from build123d import *

# Parameters (mm, degrees)
F1_DEPTH  = 90
F2_T      = -1.5
F4_DEPTH  = 90.001
F6_DEPTH  = 90
F8_DEPTH  = 90
F9_R      = 0.74999
F10_R     = 0.3
F11_DEPTH = 90.001


# Not quite as in the source:
# - a fillet or chamfer is up to 0.001 mm smaller than in the source, because OpenCascade refuses the exact size


with BuildPart() as f1:
    # F0 (on Front) → F1 (new body)
    with BuildSketch(Plane.XZ):
        with BuildLine():
            Line((40, 5), (0, 5))
            Line((0, 5), (-40, 5))
            ThreePointArc((-40, 5), (-43.3649329819, 4.389821285), (-46.301369863, 2.6369863014))
            ThreePointArc((-46.301369863, 2.6369863014), (-47.1862826711, 1.4483103051), (-47.5, 0))
            ThreePointArc((-47.5, 0), (-47.1862826711, -1.4483103051), (-46.301369863, -2.6369863014))
            ThreePointArc((-46.301369863, -2.6369863014), (-43.3649329819, -4.389821285), (-40, -5))
            Line((-40, -5), (0, -5))
            Line((0, -5), (40, -5))
            ThreePointArc((40, -5), (43.3649329819, -4.389821285), (46.301369863, -2.6369863014))
            ThreePointArc((46.301369863, -2.6369863014), (47.1862826711, -1.4483103051), (47.5, 0))
            ThreePointArc((47.5, 0), (47.1862826711, 1.4483103051), (46.301369863, 2.6369863014))
            ThreePointArc((46.301369863, 2.6369863014), (43.3649329819, 4.389821285), (40, 5))
        make_face()
    extrude(amount=F1_DEPTH)

    # F2
    f2_openings = [f1.faces().sort_by_distance(p)[0] for p in [
        (0, -90, 0),
        (0, 0, 0),
    ]]
    offset(amount=F2_T, openings=f2_openings)

    # F3 (on Front) → F4 (cut, through all)
    with BuildSketch(Plane.XZ):
        Polygon((-44, 0), (44, 0), (52.7272727273, 10), (-47.5, 10), (-47.5, -4.0104166667), align=None)
    extrude(amount=F4_DEPTH, mode=Mode.SUBTRACT)

    # F5 (on Front) → F6 (join, through all)
    with BuildSketch(Plane.XZ):
        with BuildLine():
            ThreePointArc((-40, 3.5), (-42.8382478195, 2.9853275187), (-45.3150684932, 1.5068493151))
            ThreePointArc((-45.3150684932, 1.5068493151), (-46, 0), (-45.3150684932, -1.5068493151))
            ThreePointArc((-45.3150684932, -1.5068493151), (-42.8382478195, -2.9853275187), (-40, -3.5))
            Line((-40, -3.5), (-40, -0.75))
            Line((-40, -0.75), (-34, -0.75))
            Line((-34, -0.75), (-34, 0.75))
            Line((-34, 0.75), (-40, 0.75))
            Line((-40, 0.75), (-40, 3.5))
        make_face()
    extrude(amount=F6_DEPTH)

    # F7 (on Front) → F8 (join, through all)
    with BuildSketch(Plane.XZ):
        Polygon((-16, -0.75), (-16, -3.5), (-14.5, -3.5), (-14.5, -0.75), (-9.25, -0.75), (-9.25, 0.75), (-21.25, 0.75), (-21.25, -0.75), align=None)
    extrude(amount=F8_DEPTH)

    # F9 (radius 0.75 in the source; OpenCascade refuses exactly that, so slightly less here)
    f9_edges = [f1.edges().sort_by_distance(p)[0] for p in [
        (-34, -45, 0.75),
        (-34, -45, -0.75),
        (-9.25, -45, 0.75),
        (-9.25, -45, -0.75),
        (-21.25, -45, 0.75),
        (-21.25, -45, -0.75),
    ]]
    fillet(f9_edges, radius=F9_R)

    # F10 (on Front) → F11 (cut, through all)
    with BuildSketch(Plane.XZ):
        with Locations((40, -5)):
            Circle(F10_R)
        with Locations((35, -5)):
            Circle(F10_R)
        with Locations((30, -5)):
            Circle(F10_R)
        with Locations((25, -5)):
            Circle(F10_R)
        with Locations((20, -5)):
            Circle(F10_R)
        with Locations((15, -5)):
            Circle(F10_R)
        with Locations((10, -5)):
            Circle(F10_R)
        with Locations((5, -5)):
            Circle(F10_R)
        with Locations((0, -5)):
            Circle(F10_R)
        with Locations((46.301369863, -2.6369863014)):
            Circle(F10_R)
        with Locations((-5, -5)):
            Circle(F10_R)
        with Locations((-10, -5)):
            Circle(F10_R)
        with Locations((-15, -5)):
            Circle(F10_R)
        with Locations((-20, -5)):
            Circle(F10_R)
        with Locations((-25, -5)):
            Circle(F10_R)
        with Locations((-30, -5)):
            Circle(F10_R)
        with Locations((-35, -5)):
            Circle(F10_R)
        with Locations((-40, -5)):
            Circle(F10_R)
        with Locations((46.301369863, 2.6369863014)):
            Circle(F10_R)
        with Locations((-46.301369863, -2.6369863014)):
            Circle(F10_R)
    extrude(amount=F11_DEPTH, mode=Mode.SUBTRACT)


solid = f1.part
Verification items for the finished model (mm, model axes). A direction names the side the tool comes from. Give positions to 0.01 mm unless a question says otherwise; leave off trailing zeros. Write each loop counter-clockwise with the first axis right and the second up, starting at its lowest first coordinate (ties: lowest second). Pieces come first, ordered by that corner, then holes. Notation, with made-up numbers: M 67,-26 L 101,-26 A23 cw 101,-9 Z; hole C 58,61 d8. An arc over 180 degrees is marked long. Put each result on its own line as item: value. Start each with the question number.
1. Set-up check for faces 1 (the face through (-37, -44, -0.75)), 2 (the face through (43.324, -44.37, -4.405)): record each of +Z, -Z, +X, -X, +Y, -Y from which the full face is reachable in a straight line by a thin tool's end or side.
2. Section check A-A (x = 2.5). Record the cut outline in (y, z), and give its area (3 significant figures).
3. Scan lines: line 1 along X through (y, z) = (-77, -0.5); line 2 along X through (y, z) = (-43, 0.25); line 3 along Z through (x, y) = (-24.5, -67). Record each from-to range of solid material in increasing order. Write a range as [from, to].
4. Go/stop test with flat-tipped pins: pin 1 Ø3 at (y, z) = (-62.5, 3) entering from +X; pin 2 Ø3 at (y, z) = (-44.5, -2.5) entering from +X; pin 3 Ø4 at (x, y) = (30.5, -14.5) entering from +Z. Record where each tip stops, or that it passes through.
5. Draft check along X on faces 3 (the face through (42.8, -44.4, -3)), 4 (the face through (-15, -44, 0.75)), 5 (the face through (-8, -44, -5)), 6 (the face through (-43.406, -44.37, -4.374)). Enter one of: +X half, -X half, draft (parallel to the pull), parting line (faces both ways), or undercut.
Answer list:
1. face 1: +Y, -Y
1. face 2: -Z, +X, +Y, -Y
2. outline: M -90,-5 L 0,-5 L 0,-3.5 L -90,-3.5 Z
2. area: 135 mm2
3. line 1: [-45.94, -34.19], [-21.06, -9.44], [45.94, 47.46]
3. line 2: [-45.98, -34.04], [-21.21, -9.29], [45.98, 47.49]
3. line 3: [-5, -3.5]
4. pin 1: x = 47.16
4. pin 2: x = 47.35
4. pin 3: z = -3.5
5. face 3: undercut
5. face 4: undercut
5. face 5: draft
5. face 6: -X half
